from build123d import *

# Parameters (mm, degrees)
SKETCH1_W           = 13.6
SKETCH1_H           = 12.5
BOSS_EXTRUDE1_DEPTH = 1
SKETCH2_W           = 7
SKETCH2_H           = 7
BOSS_EXTRUDE2_DEPTH = 1
SKETCH3_W           = 3.3
SKETCH3_H           = 2.6
BOSS_EXTRUDE3_DEPTH = 1
FILLET1_R           = 0.1


with BuildPart() as part:
    # Sketch1 → Boss-Extrude1 (new body)
    with BuildSketch(Plane(origin=(0, 0, 0), x_dir=(1, 0, 0), z_dir=(0, 1, 0))):
        Rectangle(SKETCH1_W, SKETCH1_H)
    extrude(amount=BOSS_EXTRUDE1_DEPTH)

    # Sketch2 → Boss-Extrude2 (add)
    with BuildSketch(Plane(origin=(0, 1, 0), x_dir=(1, 0, 0), z_dir=(0, 1, 0))):
        with Locations((2.1, -1.75)):
            Rectangle(SKETCH2_W, SKETCH2_H)
    extrude(amount=BOSS_EXTRUDE2_DEPTH)

    # Sketch3 → Boss-Extrude3 (add)
    with BuildSketch(Plane(origin=(0, 1, 0), x_dir=(1, 0, 0), z_dir=(0, 1, 0))):
        with Locations((-2.85, 3.85)):
            Rectangle(SKETCH3_W, SKETCH3_H)
    extrude(amount=BOSS_EXTRUDE3_DEPTH)

    # Fillet1
    fillet1_edges = [part.edges().sort_by_distance(p)[0] for p in [
        (6.8, 1, 0),
        (0, 1, -6.25),
        (-4.5, 1, -3.85),
        (-4.5, 1.5, -5.15),
        (-2.85, 1, -2.55),
        (-4.5, 1.5, -2.55),
        (-1.2, 1, -3.85),
        (-1.2, 1.5, -2.55),
        (-2.85, 1, -5.15),
        (-1.2, 1.5, -5.15),
        (-4.5, 2, -3.85),
        (-2.85, 2, -2.55),
        (-1.2, 2, -3.85),
        (-2.85, 2, -5.15),
        (-6.8, 1, 0),
        (0, 1, 6.25),
        (-6.8, 0.5, -6.25),
        (6.8, 0.5, -6.25),
        (6.8, 0.5, 6.25),
        (-6.8, 0.5, 6.25),
    ]]
    fillet(fillet1_edges, radius=FILLET1_R)


solid = part.part
Check sheet for the modelled part. Datum: model origin and axes. Units: mm. A direction names the side the tool comes from. Round coordinates to 2 decimals unless told otherwise and drop trailing zeros. Write each loop counter-clockwise with the first axis right and the second up, starting at its lowest first coordinate (ties: lowest second). Pieces come first, ordered by that corner, then holes. Notation, with made-up numbers: (66.5, -1) - (106.5, -1) arc R21 cw to (106.5, 14) - close; hole circle Ø10 at (57, 18). An arc over 180 degrees is marked (long way). Return JSON: item names as keys, results as strings.
Q1. Cross-section at B-B (x = -2.75). Record the boundary of the cut face in (y, z).
Returned:
{"outline": "(0, -6.25) - (0.9, -6.25) arc R0.1 ccw to (1, -6.15) - (1, -5.25) arc R0.1 cw to (1.1, -5.15) - (1.9, -5.15) arc R0.1 ccw to (2, -5.05) - (2, -2.65) arc R0.1 ccw to (1.9, -2.55) - (1.1, -2.55) arc R0.1 cw to (1, -2.45) - (1, 6.15) arc R0.1 ccw to (0.9, 6.25) - (0, 6.25) - close"}
Q2. Cross-section at C-C (z = 0). Record the boundary of the cut face in (x, y), then the cut area to 3 significant figures.
Returned:
{"outline": "(-6.8, 0) - (6.8, 0) - (6.8, 0.9) arc R0.1 ccw to (6.7, 1) - (5.6, 1) - (5.6, 2) - (-1.4, 2) - (-1.4, 1) - (-6.7, 1) arc R0.1 ccw to (-6.8, 0.9) - close", "area": "20.6 mm²"}
Q3. Cross-section at A-A (y = 1.45). Record the boundary of the cut face in (x, z).
Returned:
{"outline": "(-4.5, -5.05) arc R0.1 ccw to (-4.4, -5.15) - (-1.3, -5.15) arc R0.1 ccw to (-1.2, -5.05) - (-1.2, -2.65) arc R0.1 ccw to (-1.3, -2.55) - (-4.4, -2.55) arc R0.1 ccw to (-4.5, -2.65) - close; (-1.4, -1.75) - (5.6, -1.75) - (5.6, 5.25) - (-1.4, 5.25) - close"}
Q4. Scan lines: L1, parallel to Y at x = -5, z = 3.25; L2, parallel to X at y = 1.25, z = -4.25; L3, parallel to Z at x = -0.75, y = 1.75. Record each from-to range of solid material in increasing order. Write a range as from..to.
Returned:
{"L1": "y = 0..1", "L2": "x = -4.5..-1.2", "L3": "z = -1.75..5.25"}
Q5. Cross-section at D-D (x = 5.25). Record the boundary of the cut face in (y, z).
Returned:
{"outline": "(0, -6.25) - (0.9, -6.25) arc R0.1 ccw to (1, -6.15) - (1, -1.75) - (2, -1.75) - (2, 5.25) - (1, 5.25) - (1, 6.15) arc R0.1 ccw to (0.9, 6.25) - (0, 6.25) - close"}
Q6. Depth check by flat-ended pin: P1, Ø0.5, axis at x = 1.5, y = 1.5, coming from the +Z side; P2, Ø0.5, axis at y = 1.5, z = 3, coming from the +X side; P3, Ø0.5, axis at x = 3.5, y = 1.5, coming from the -Z side. Enter the tip coordinate at first touch or a pass-through.
Returned:
{"P1": "stops at z = 5.25", "P2": "stops at x = 5.6", "P3": "stops at z = -1.75"}
Q7. Access from +Z, -Z, +X, -X, +Y, -Y to the whole of each face (thin tool, end or side, straight path). Record for faces 1 (the flat face through (2.1, 1.5, 5.25)), 2 (the flat face through (-1.4, 1.5, 1.8)), 3 (the flat face through (5.6, 1.5, 1.8)).
Returned:
{"face 1": "+Z, +X, -X, +Y", "face 2": "+Z, -X, +Y", "face 3": "+Z, -Z, +X, +Y"}
